from build123d import *

# Parameters (mm, degrees)
F1_DEPTH = 25
F2_R     = 62.8315
F3_DEPTH = 16.6
F5_DEPTH = 50


with BuildPart() as f1:
    # F0 (on Front) → F1 (new body)
    with BuildSketch(Plane.XZ):
        Polygon((-74.484, 0), (0, 0), (-37.114122, 64.578698), align=None)
        Polygon((-37.114122, 64.578698), (0, 0), (37.114122, 64.578698), align=None)
        Polygon((37.114122, 64.578698), (0, 0), (74.484, 0), align=None)
        Polygon((74.484, 0), (0, 0), (37.369732, -64.431121), align=None)
        Polygon((37.369732, -64.431121), (0, 0), (-37.242, -64.505036), align=None)
        Polygon((-37.242, -64.505036), (0, 0), (-74.484, 0), align=None)
    extrude(amount=F1_DEPTH)

    # F2 (on face) → F3 (cut)
    with BuildSketch(Plane.XZ.offset(25)):
        Circle(F2_R)
    extrude(amount=-F3_DEPTH, mode=Mode.SUBTRACT)

    # F4 (on face) → F5 (join)
    with BuildSketch(Plane.XZ.offset(8.4)):
        with BuildLine():
            ThreePointArc((-11.518612, 30.355605), (15.876825, 35.305832), (38.545772, 19.146203))
            ThreePointArc((38.545772, 19.146203), (24.321415, 41.530617), (-1.657793, 46.866823))
            Line((-1.657793, 46.866823), (-11.518612, 30.355605))
        make_face()
    extrude(amount=F5_DEPTH)


solid = f1.part
Can you work these out from the model? Positions are in its coordinate system, mm. A direction names the side the tool comes from. Coordinates: 2 decimals unless noted, no trailing zeros. Write each loop counter-clockwise with the first axis right and the second up, starting at its lowest first coordinate (ties: lowest second). Pieces come first, ordered by that corner, then holes. Notation, with made-up numbers: M 1.5,-30.5 L 48.5,-30.5 A9 cw 48.5,-22.5 Z; hole C 65,11.25 d8. An arc over 180 degrees is marked long. Use one line per item in the form item = value.
Q1. If we section it at D-D (y = -31): Write out the boundary of the cut face in (x, z).
Model answer:
outline = M -11.52,30.36 A35.83 cw 38.55,19.15 A33.97 ccw -1.66,46.87 Z
Q2. If we section it at C-C (z = -22): Write out the boundary of the cut face in (x, y).
Model answer:
outline = M -61.78,-25 L -58.85,-25 L -58.85,-8.4 L 58.85,-8.4 L 58.85,-25 L 61.81,-25 L 61.81,0 L -61.78,0 Z
Q3. If we section it at B-B (x = 48.5): Write out the boundary of the cut face in (y, z).
Model answer:
outline = M -25,-45.11 L 0,-45.11 L 0,44.9 L -25,44.9 L -25,39.94 L -8.4,39.94 L -8.4,-39.94 L -25,-39.94 Z
Q4. We'd pull the mould along Z, two halves only. Please class faces 3 (the flat face through (13, -58.4, 38)), 4 (the cylindrical face through (-13.621, -16.816, -61.337)), 5 (the cylindrical face through (15.49, -33.05, 35.39)), 6 (the flat face through (-56.124, -12.325, -31.801)): +Z half, -Z half, draft (parallel to the pull), parting line (faces both ways), or undercut.
Model answer:
face_3 = draft
face_4 = undercut
face_5 = undercut
face_6 = -Z half
Q5. For P1, Ø1, axis at y = -7, z = -16.5, coming from the -X side; P2, Ø1, axis at x = 52, y = -11.5, coming from the +Z side; P3, Ø12, axis at x = 30.5, z = -14.5, coming from the -Y side, each with a flat end and sliding along its axis, tell me the tip position at first contact or that it passes through.
Model answer:
P1 = -65.25
P2 = 39.72
P3 = -8.4
Q6. I need wall thicknesses on line 1 along Z through (x, y) = (0, -14); line 2 along Z through (x, y) = (17, -23); line 3 along Y through (x, z) = (-15.5, 11). Which ranges of each line are inside material? Lowest first, please. Write a range as from..to.
Model answer:
line_1 = -64.47..-62.83, 35.26..47.16, 62.83..64.58
line_2 = -64.45..-60.49, 35.04..45.36, 60.49..64.58
line_3 = -8.4..0
Q7. If we section it at A-A (y = -19): Write out the boundary of the cut face in (x, z).
Model answer:
outline = M -74.48,0 L -37.24,-64.51 L 37.37,-64.43 L 74.48,0 L 37.11,64.58 L -37.11,64.58 Z; M -11.52,30.36 A35.83 cw 38.55,19.15 A33.97 ccw -1.66,46.87 Z; hole C 0,0 d125.66
Q8. For faces 1 (the flat face through (1, -12, 64.579)), 2 (the cylindrical face through (24.634, -33.05, 41.312)), which set-ups out of +Z, -Z, +X, -X, +Y, -Y let a thin tool reach every point of the face, with its end or its side?
Model answer:
face_1 = +Z, +X, -X, +Y, -Y
face_2 = -Y
